Verification items for the finished model (mm, model axes). A direction names the side the tool comes from. Coordinates: 2 decimals unless noted, no trailing zeros. Order: outer loops, then holes, each group sorted by start corner. A loop starts at its lowest first (then second) coordinate and runs counter-clockwise, first axis right, second up. Notation, with made-up numbers: (50.5, 25) -> (97.5, 25) arc R21 ccw to (97.5, 32) -> close; hole circle Ø10 at (27, 34). An arc over 180 degrees is marked (long way). Use CSV: the item, a comma, the result in double quotes. Start each with the question number.
1) Release check for a two-part mould opening along X. For faces 1 (the cylindrical face through (-3.252, -14.643, -0.454)), 2 (the flat face through (0, 0, -40)), 3 (the flat face through (0, 13, -20)) record: released by +X, released by -X, zero draft, split by the parting line, or undercut.
2) Scan lines: line 1 along Y through (x, z) = (-0.5, 25); line 2 along Z through (x, y) = (-1, 13.25); line 3 along Y through (x, z) = (7.5, 31). Record each from-to range of solid material in increasing order.
3) Sectioned sample at A-A on x = 0. Record the boundary of the cut face in (y, z), then the cut area to 3 significant figures.
4) Go/stop test with flat-tipped pins: pin 1 (4 mm diameter, centred on x = -7, z = 20.5, fed in from -Y); pin 2 (4 mm diameter, centred on x = -3.5, z = -15.5, fed in from +Y); pin 3 (8 mm diameter, centred on y = -5, z = 17.5, fed in from -X). Record where each tip stops, or that it passes through.
5) Sectioned sample at B-B on z = 11. Record the boundary of the cut face in (x, y).
6) Tool access check on faces 4 (the conical face through (-0.54, -13.31, 39.68)), 5 (the flat face through (0, 11, 10)). Record the directions out of +Z, -Z, +X, -X, +Y, -Y that give a thin tool (end or side, any length) a straight path to the whole face; none if there is none.
from build123d import *

# Parameters (mm, degrees)
SKETCH1_R           = 15
BOSS_EXTRUDE1_DEPTH = 40
CUT_EXTRUDE1_DEPTH  = 60
CHAMFER1_SIZE       = 2


with BuildPart() as part:
    # Sketch1 → Boss-Extrude1 (new, symmetric)
    with BuildSketch(Plane.XY):
        Circle(SKETCH1_R)
    extrude(amount=BOSS_EXTRUDE1_DEPTH, both=True)

    # Sketch2 → Cut-Extrude1 (cut)
    with BuildSketch(Plane.XY.offset(40)):
        with BuildLine():
            Line((-4, 14.456832295), (-4, 11))
            Line((-4, 11), (4, 11))
            Line((4, 11), (4, 14.456832295))
            ThreePointArc((4, 14.456832295), (0, 15), (-4, 14.456832295))
        make_face()
    extrude(amount=-CUT_EXTRUDE1_DEPTH, mode=Mode.SUBTRACT)

    # Chamfer1
    chamfer1_edges = [part.edges().sort_by_distance(p)[0] for p in [
        (-9.082951062, -11.937336386, 40),
    ]]
    chamfer(chamfer1_edges, length=CHAMFER1_SIZE)


solid = part.part
Answers follow:
1,face 1,"split by the parting line"
1,face 2,"zero draft"
1,face 3,"undercut"
2,line 1,"y = -14.99 to 11"
2,line 2,"z = -40 to -20"
2,line 3,"y = -12.99 to 12.99"
3,outline,"(-15, -40) -> (15, -40) -> (15, -20) -> (11, -20) -> (11, 40) -> (-13, 40) -> (-15, 38) -> close"
3,area,"2,160 mm²"
4,pin 1,"stops at y = -14.14"
4,pin 2,"stops at y = 14.46"
4,pin 3,"stops at x = -14.97"
5,outline,"(-4, 11) -> (-4, 14.46) arc R15 ccw (long way) to (4, 14.46) -> (4, 11) -> close"
6,face 4,"+Z"
6,face 5,"+Z, +Y"
